CAD build for the part. Positions are in the model's coordinates, mm. Face numbers are marked on the shaded views. Round coordinates to 2 decimals unless told otherwise and drop trailing zeros. Write each loop counter-clockwise with the first axis right and the second up, starting at its lowest first coordinate (ties: lowest second). Pieces come first, ordered by that corner, then holes. Notation, with made-up numbers: (56.25, 0.5) - (82.25, 0.5) arc R15 cw to (82.25, 7.5) - close; hole circle Ø10 at (0, 37). An arc over 180 degrees is marked (long way). Use one line per item in the form item = value. Start each with the question number.
Item 1: Pull direction Y, two halves, no side cores. Call the marked faces 1, 2 and 3: +Y half, -Y half, draft (parallel to the pull), parting line (faces both ways), or undercut.
Item 2: Drill centre lines: L1, parallel to Y at x = 11, z = 2.75; L2, parallel to Z at x = -0.5, y = -66.5; L3, parallel to X at y = -9, z = 2.5. Where is each one in solid material? Low to high.
Item 3: Band-saw the part on B-B, the plane y = -44.5. List the corners of the cut face in (x, z) (3 decimals), and give its area (3 significant figures).
Item 4: Band-saw the part on C-C, the plane x = -9. List the corners of the cut face in (y, z), and give its area (3 significant figures).
Item 5: Band-saw the part on A-A, the plane x = -1.5. List the corners of the cut face in (y, z).
Item 6: Pin check, flat tips, straight feed: pin 1 (1.9 mm diameter, centred on y = -58, z = -0.5, fed in from -X); pin 2 (3 mm diameter, centred on x = -2, y = -39.5, fed in from -Z); pin 3 (5 mm diameter, centred on x = -10, y = -62.5, fed in from +Z); pin 4 (2 mm diameter, centred on x = 2.5, y = -69, fed in from -Z). Stop position of each tip, or through.
from build123d import *

# Parameters (mm, degrees)
BOSS_EXTRUDE1_DEPTH = 101.6
BOSS_EXTRUDE3_DEPTH = 12.7


with BuildPart() as part:
    # Sketch1 → Boss-Extrude1 (new body)
    with BuildSketch(Plane(origin=(0, 0, 0), x_dir=(1, 0, 0), z_dir=(0, 1, 0))):
        with BuildLine():
            Line((-5.499261314, 3.175), (-5.499261314, -3.175))
            ThreePointArc((-5.499261314, -3.175), (1.643500936, -6.133628997), (6.35, 0))
            ThreePointArc((6.35, 0), (1.643500936, 6.133628997), (-5.499261314, 3.175))
        make_face()
    extrude(amount=-BOSS_EXTRUDE1_DEPTH)

    # Sketch4 → Boss-Extrude3 (add)
    with BuildSketch(Plane(origin=(0, 0, 0), x_dir=(1, 0, 0), z_dir=(0, 1, 0))):
        with BuildLine():
            Line((-6.35, 6.35), (6.35, 6.35))
            ThreePointArc((6.35, 6.35), (12.7, 0), (6.35, -6.35))
            Line((6.35, -6.35), (-6.35, -6.35))
            ThreePointArc((-6.35, -6.35), (-12.7, 0), (-6.35, 6.35))
        make_face()
    extrude(amount=BOSS_EXTRUDE3_DEPTH)


solid = part.part
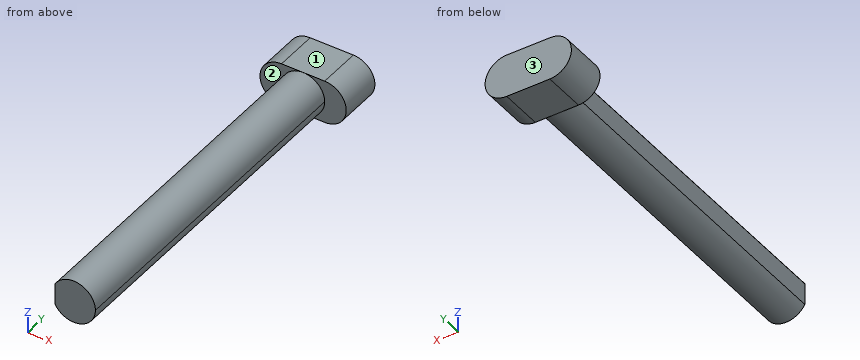
Determined:
q1.face_1 = draft
q1.face_2 = -Y half
q1.face_3 = +Y half
q2.L1 = 0 to 12.7
q2.L2 = -6.33 to 6.33
q2.L3 = -5.5 to 5.84
q3.outline = (-5.499, -3.175) arc R6.35 ccw (long way) to (-5.499, 3.175) - close
q3.area = 123 mm²
q4.outline = (0, -5.77) - (12.7, -5.77) - (12.7, 5.77) - (0, 5.77) - close
q4.area = 147 mm²
q5.outline = (-101.6, -6.17) - (0, -6.17) - (0, -6.35) - (12.7, -6.35) - (12.7, 6.35) - (0, 6.35) - (0, 6.17) - (-101.6, 6.17) - close
q6.pin_1 = -5.5
q6.pin_2 = -6.33
q6.pin_3 = through
q6.pin_4 = -6.17
